from build123d import *

# Parameters (mm, degrees)
F1_DEPTH = 25


with BuildPart() as f1:
    # F0 (on Top) → F1 (new body)
    with BuildSketch(Plane.XY):
        Polygon((-59.6113632321, -28.6996493522), (-25, -25), (-25, 25), (-59.6113632321, 28.6996493522), (-76.1811135112, 0), align=None)
        Polygon((-9.9021123947, 0), (-24.3358691244, -25), (24.3358691244, -25), (9.9021123947, 0), (24.3358691244, 25), (-24.3358691244, 25), align=None)
        Polygon((-25, 25), (-25, -25), (-24.3358691244, -25), (-9.9021123947, 0), (-24.3358691244, 25), align=None)
        Polygon((9.9021123947, 0), (24.3358691244, -25), (25, -25), (25, 25), (24.3358691244, 25), align=None)
        Polygon((25, 25), (25, -25), (59.6113632321, -28.6996493522), (76.1811135112, 0), (59.6113632321, 28.6996493522), align=None)
    extrude(amount=F1_DEPTH)


solid = f1.part
The listing builds one solid part. Answer for the finished solid, in the listing's coordinates (mm). A direction names the side the tool comes from. Give positions to 0.01 mm unless a question says otherwise; leave off trailing zeros. Write each loop counter-clockwise with the first axis right and the second up, starting at its lowest first coordinate (ties: lowest second). Pieces come first, ordered by that corner, then holes.
1) Section B-B (x = -23) is taken. Write down the section's boundary in (y, z).
2) Given P1, Ø4, axis at x = 42.5, y = 17, coming from the -Z side; P2, Ø4, axis at x = -5.5, z = 13.5, coming from the -Y side; P3, Ø12, axis at y = 14.5, z = 19.5, coming from the +X side; P4, Ø1.5, axis at y = -1, z = 7.5, coming from the -X side, each flat-ended and moving along its own axis, determine where each tip first touches the part or whether it passes through.
3) Section A-A (z = 3) is taken. Write down the section's boundary in (x, y).
4) A tool of negligible diameter and unlimited length cuts with its end or side. For faces 1 (the face through (42.063, -26.824, 12.325)), 2 (the face through (42.548, 26.876, 12.325)), 3 (the face through (67.78, -14.55, 12.32)), from which of +Z, -Z, +X, -X, +Y, -Y can it reach the whole face along a straight path? Write none if from no direction.
5) Section C-C (y = 2.5) is taken. Write down the section's boundary in (x, z).
6) Find the intervals of material crossed by L1, parallel to Y at x = 25, z = 1; L2, parallel to Y at x = 49.5, z = 20.5; L3, parallel to X at y = -17, z = 5, in increasing order.
Response:
1. outline: (-25, 0) - (25, 0) - (25, 25) - (-25, 25) - close
2. P1: stops at z = 0
2. P2: stops at y = -25
2. P3: stops at x = 71.27
2. P4: stops at x = -76.04
3. outline: (-76.18, 0) - (-59.61, -28.7) - (-25, -25) - (25, -25) - (59.61, -28.7) - (76.18, 0) - (59.61, 28.7) - (25, 25) - (-25, 25) - (-59.61, 28.7) - close
4. face 1: +Z, -Z, -Y
4. face 2: +Z, -Z, +Y
4. face 3: +Z, -Z, +X, -Y
5. outline: (-74.74, 0) - (74.74, 0) - (74.74, 25) - (-74.74, 25) - close
6. L1: y = -25 to 25
6. L2: y = -27.62 to 27.62
6. L3: x = -66.37 to 66.37
